Design review of the part built by this model. Coordinates are the model's own, in mm. A direction names the side the tool comes from. Coordinates: 2 decimals unless noted, no trailing zeros. Loops run counter-clockwise (first coordinate to the right, second up) from the corner with the lowest first, then second, coordinate; pieces in that order, holes last. Notation, with made-up numbers: (-5, 28) - (35, 28) arc R18 ccw to (35, 62) - close; hole circle Ø2 at (77, 40). An arc over 180 degrees is marked (long way). Use one line per item in the form item = value. Start each with the question number.
(1) Add section D-D (y = 19.5). State the section outline as (x, z) points.
(2) Clearance check with flat-ended pins moving along their axes: pin 1 Ø1.6 at (x, y) = (-1, 18) entering from +Z; pin 2 Ø2.5 at (x, z) = (-10, 2) entering from -Y; pin 3 Ø5 at (y, z) = (1, 4.5) entering from -X; pin 4 Ø8 at (x, y) = (-12.5, -2) entering from -Z. State where each tip first meets the part, or that it passes through.
(3) Add section B-B (y = 10). State the section outline as (x, z) points, plus the area to 3 significant figures.
(4) Add section A-A (x = -15). State the section outline as (y, z) points.
(5) Add section C-C (z = 5). Count the separate pieces of the cut face and the enclosed holes in it, plus the area to 3 significant figures.
(6) The part is to be moulded in two halves that separate along Z. For faces 1 (the face through (-0.358, 22.227, 8.521)), 2 (the face through (0.07, -8.464, 5.325)), 3 (the face through (-4.5, 5.2, 0)), say which applies: pulls with the +Z half, pulls with the -Z half, needs draft (parallel to the pull), parting line crosses it, or undercut.
(7) Tool access review of faces 4 (the face through (-4.57, 24.55, 6.55)), 5 (the face through (5, 3, 5)), 6 (the face through (-4.3, 25, 2.7)), 7 (the face through (2, 20, 7)), 8 (the face through (-11, 15, 1)): name each direction out of +Z, -Z, +X, -X, +Y, -Y from which nothing blocks a thin tool from reaching the whole face with its end or side.
(8) For L1, parallel to Y at x = -15, z = 1.65; L2, parallel to Y at x = 4.25, z = 5.5; L3, parallel to Y at x = -0.5, z = 5.5, list the stretches that pass through material, from the lowest coordinate up.
```python
from build123d import *

# Parameters (mm, degrees)
SKETCH1_W           = 10
SKETCH1_H           = 50
BOSS_EXTRUDE1_DEPTH = 10
SKETCH2_R           = 1.75
CUT_EXTRUDE1_DEPTH  = 10
CUT_EXTRUDE2_DEPTH  = 10
FILLET1_R           = 1.5
SKETCH4_R           = 2.75
CUT_EXTRUDE3_DEPTH  = 3
SKETCH5_R           = 3
CUT_EXTRUDE4_DEPTH  = 13
SKETCH6_W           = 3
SKETCH6_H           = 10
BOSS_EXTRUDE2_DEPTH = 15
FILLET2_R           = 3
FILLET3_R           = 1.5
SKETCH7_R           = 1.35
CUT_EXTRUDE5_DEPTH  = 15
SKETCH8_R           = 1.5
CUT_EXTRUDE6_DEPTH  = 15


with BuildPart() as part:
    # Sketch1 → Boss-Extrude1 (new body)
    with BuildSketch(Plane.XY):
        Rectangle(SKETCH1_W, SKETCH1_H)
    extrude(amount=BOSS_EXTRUDE1_DEPTH)

    # Sketch2 → Cut-Extrude1 (cut)
    with BuildSketch(Plane.XY.offset(10)):
        with Locations((0, 19.5)):
            Circle(SKETCH2_R)
    extrude(amount=-CUT_EXTRUDE1_DEPTH, mode=Mode.SUBTRACT)

    # Sketch3 → Cut-Extrude2 (cut)
    with BuildSketch(Plane.XY.offset(10)):
        with BuildLine():
            Line((5, -18), (5, -25))
            Line((5, -25), (-2, -25))
            add(Edge.make_bspline(
                [(-2, -25), (-1.904224842, -19.430935455), (5, -18)],
                knots=[0, 0, 0, 1, 1, 1], degree=2))
        make_face()
    extrude(amount=-CUT_EXTRUDE2_DEPTH, mode=Mode.SUBTRACT)

    # Fillet1
    fillet1_edges = [part.edges().sort_by_distance(p)[0] for p in [
        (5, -18, 5),
        (-2, -25, 5),
        (-5, -25, 5),
        (5, 25, 5),
    ]]
    fillet(fillet1_edges, radius=FILLET1_R)

    # Sketch4 → Cut-Extrude3 (cut)
    with BuildSketch(Plane.XY.offset(10)):
        with Locations((0, 19.5)):
            Circle(SKETCH4_R)
    extrude(amount=-CUT_EXTRUDE3_DEPTH, mode=Mode.SUBTRACT)

    # Sketch5 → Cut-Extrude4 (cut)
    with BuildSketch(Plane(origin=(5, 0, 0), x_dir=(0, 0, -1), z_dir=(1, 0, 0))):
        with Locations((-5, 10)):
            Circle(SKETCH5_R)
    extrude(amount=-CUT_EXTRUDE4_DEPTH, mode=Mode.SUBTRACT)

    # Sketch6 → Boss-Extrude2 (add)
    with BuildSketch(Plane.ZY.offset(5)):
        with Locations((1.5, 20)):
            Rectangle(SKETCH6_W, SKETCH6_H)
    extrude(amount=BOSS_EXTRUDE2_DEPTH)

    # Fillet2
    fillet2_edges = [part.edges().sort_by_distance(p)[0] for p in [
        (-20, 15, 1.5),
        (-20, 25, 1.5),
    ]]
    fillet(fillet2_edges, radius=FILLET2_R)

    # Fillet3
    fillet3_edges = [part.edges().sort_by_distance(p)[0] for p in [
        (-5, 25, 6.5),
    ]]
    fillet(fillet3_edges, radius=FILLET3_R)

    # Sketch7 → Cut-Extrude5 (cut)
    with BuildSketch(Plane.XY.offset(3)):
        with Locations((-15, 19.5)):
            Circle(SKETCH7_R)
    extrude(amount=-CUT_EXTRUDE5_DEPTH, mode=Mode.SUBTRACT)

    # Sketch8 → Cut-Extrude6 (cut)
    with BuildSketch(Plane(origin=(5, 0, 0), x_dir=(0, 0, -1), z_dir=(1, 0, 0))):
        with Locations((-5, -7)):
            Circle(SKETCH8_R)
    extrude(amount=-CUT_EXTRUDE6_DEPTH, mode=Mode.SUBTRACT)


solid = part.part
```
Computed values:
q1.outline = (-20, 0) - (-16.35, 0) - (-16.35, 3) - (-20, 3) - close; (-13.65, 0) - (-1.75, 0) - (-1.75, 7) - (-2.75, 7) - (-2.75, 10) - (-5, 10) - (-5, 3) - (-13.65, 3) - close; (1.75, 0) - (5, 0) - (5, 10) - (2.75, 10) - (2.75, 7) - (1.75, 7) - close
q2.pin_1 = 7
q2.pin_2 = 15
q2.pin_3 = -5
q2.pin_4 = through
q3.outline = (-5, 0) - (5, 0) - (5, 2) - (-5, 2) - close; (-5, 8) - (5, 8) - (5, 10) - (-5, 10) - close
q3.area = 40.0 mm^2
q4.outline = (15, 0) - (18.15, 0) - (18.15, 3) - (15, 3) - close; (20.85, 0) - (25, 0) - (25, 3) - (20.85, 3) - close
q5.separate_pieces = 3
q5.enclosed_holes = 1
q5.area = 361 mm^2
q6.face_1 = needs draft
q6.face_2 = undercut
q6.face_3 = pulls with the -Z half
q7.face_4 = +Z, -X, +Y
q7.face_5 = +Z, -Z, +X, +Y, -Y
q7.face_6 = +Z, -Z, +X, -X, +Y
q7.face_7 = +Z
q7.face_8 = +Z, -Z, -X, -Y
q8.L1 = 15 to 18.15, 20.85 to 25
q8.L2 = -18.12 to -8.41, -5.59 to 7.04, 12.96 to 24.8
q8.L3 = -20.79 to -8.41, -5.59 to 7.04, 12.96 to 17.82, 21.18 to 25
